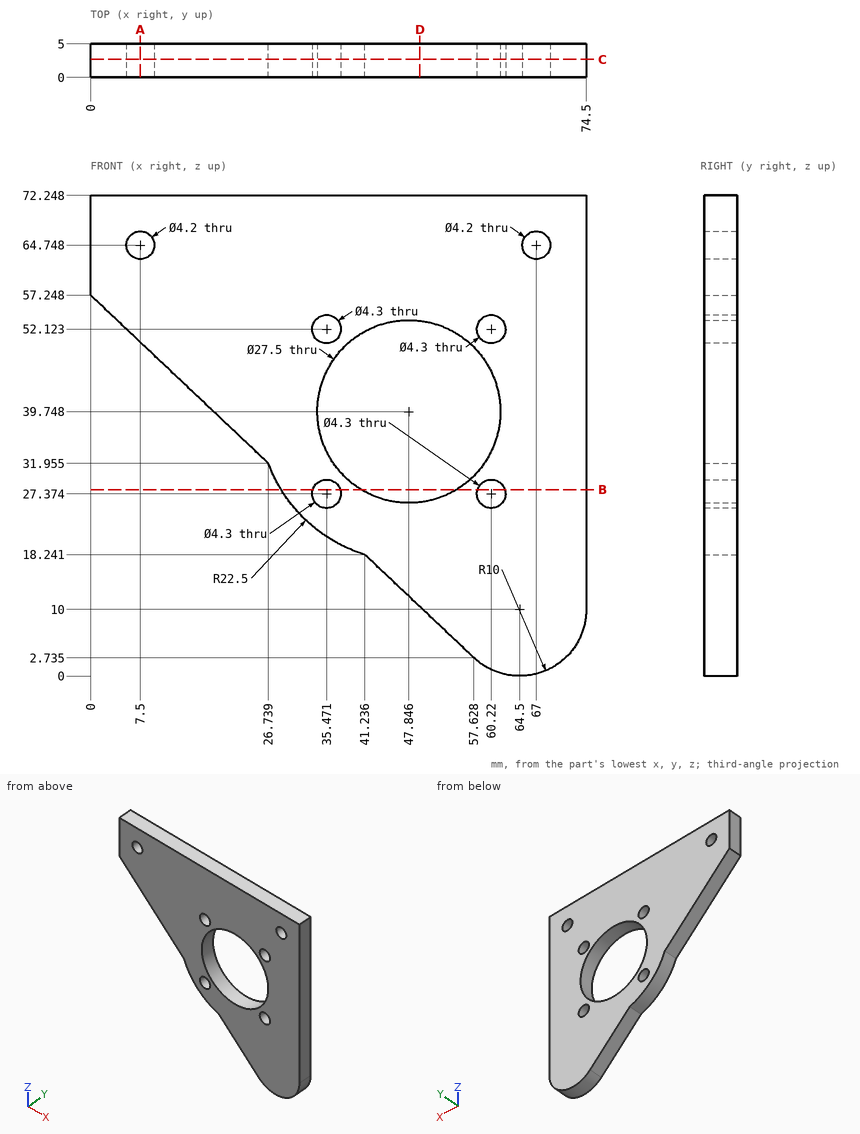
The drawing under review shows one solid part. Ordinate dimensions are in mm from its lowest x, y, z. Round coordinates to 2 decimals unless told otherwise and drop trailing zeros. Loops run counter-clockwise (first coordinate to the right, second up) from the corner with the lowest first, then second, coordinate; pieces in that order, holes last. Notation, with made-up numbers: (76, 81) - (107, 81) arc R18 ccw to (107, 106) - close; hole circle Ø10 at (-8.5, 86.5). An arc over 180 degrees is marked (long way). Use a Markdown table: item, result. Add a question column.
Q1. Add section B-B (z = 28). State the section outline as (x, y) points (1 decimal), plus the area to 3 significant figures.
Q2. Add section C-C (y = 2.7). State how many separate pieces and enclosed holes the cut face has, plus the area to 3 significant figures.
Q3. For probe 1 along X at (y, z) = (3.7, 65.5); probe 2 along X at (y, z) = (1.2, 32.5) (1 decimal); probe 3 along Z at (x, y) = (67, 1.15), list the stretches that pass through material, from the lowest coordinate up.
Q4. Insertion check: pin 1 Ø4 at (x, z) = (67, 64.75) entering from -Y; pin 2 Ø1 at (y, z) = (1, 11.5) entering from -X (1 decimal); pin 3 Ø2 at (y, z) = (3.5, 53.5) entering from -X (1 decimal); pin 4 Ø2 at (y, z) = (1.5, 43) entering from -X (1 decimal). Each pin has a flat end and moves straight along its axis. Give the tip position at first contact, or say it passes through.
Q5. Add section A-A (x = 7.5). State the section outline as (y, z) points.
Q6. Add section D-D (x = 49.5). State the section outline as (y, z) points, plus the area to 3 significant figures.
Worked answers:
| question | item | result |
|---|---|---|
| 1 | outline | (28.7, 0) - (33.4, 0) - (33.4, 5) - (28.7, 5) - close; (37.5, 0) - (40.7, 0) - (40.7, 5) - (37.5, 5) - close; (55, 0) - (58.2, 0) - (58.2, 5) - (55, 5) - close; (62.3, 0) - (74.5, 0) - (74.5, 5) - (62.3, 5) - close |
| 1 | area | 117 mm² |
| 2 | separate pieces | 1 |
| 2 | enclosed holes | 7 |
| 2 | area | 2,980 mm² |
| 3 | probe 1 | 0 to 5.54, 9.46 to 65.04, 68.96 to 74.5 |
| 3 | probe 2 | 26.2 to 36.2, 59.5 to 74.5 |
| 3 | probe 3 | 0.32 to 62.65, 66.85 to 72.25 |
| 4 | pin 1 | through |
| 4 | pin 2 | x = 47.8 |
| 4 | pin 3 | x = 2.9 |
| 4 | pin 4 | x = 14 |
| 5 | outline | (0, 50.15) - (5, 50.15) - (5, 62.65) - (0, 62.65) - close; (0, 66.85) - (5, 66.85) - (5, 72.25) - (0, 72.25) - close |
| 6 | outline | (0, 10.42) - (5, 10.42) - (5, 26.1) - (0, 26.1) - close; (0, 53.4) - (5, 53.4) - (5, 72.25) - (0, 72.25) - close |
| 6 | area | 173 mm² |
